from build123d import *

# Parameters (mm, degrees)
SKETCH1_R           = 4.25
SKETCH1_R_2         = 1.25
BOSS_EXTRUDE1_DEPTH = 3
BOSS_EXTRUDE2_START = -3
SKETCH2_R           = 2.5
SKETCH2_R_2         = 1.25
BOSS_EXTRUDE2_DEPTH = 6


with BuildPart() as part:
    # Sketch1 → Boss-Extrude1 (new body)
    # profile 1 of 4: a face of its own
    with BuildSketch(Plane(origin=(0, 0, 0), x_dir=(1, 0, 0), z_dir=(0, 1, 0))):
        with BuildLine():
            ThreePointArc((1.6e-08, -11.5), (-11.5, -2.4e-08), (-3.2e-08, 11.5))
            ThreePointArc((-3.2e-08, 11.5), (-4.157986242, 14.870426004), (-1.721061947, 19.635929204))
            ThreePointArc((-1.721061947, 19.635929204), (-14.5, 0), (-1.721061947, -19.635929204))
            ThreePointArc((-1.721061947, -19.635929204), (-4.157986237, -14.87042598), (1.6e-08, -11.5))
        make_face()
    # profile 2 of 4: a face of its own
    with BuildSketch(Plane(origin=(0, 0, 0), x_dir=(1, 0, 0), z_dir=(0, 1, 0))):
        with BuildLine():
            ThreePointArc((1.721061947, 19.635929204), (3.562093014, 18.068187517), (4.25, 15.75))
            ThreePointArc((4.25, 15.75), (3.005203809, 12.744796169), (-3.2e-08, 11.5))
            ThreePointArc((-3.2e-08, 11.5), (8.131727972, 8.131727995), (11.5, 0))
            ThreePointArc((11.5, 0), (8.131727989, -8.131727978), (1.6e-08, -11.5))
            ThreePointArc((1.6e-08, -11.5), (3.005203826, -12.744796186), (4.25, -15.75))
            ThreePointArc((4.25, -15.75), (3.562093014, -18.068187517), (1.721061947, -19.635929204))
            ThreePointArc((1.721061947, -19.635929204), (14.5, 0), (1.721061947, 19.635929204))
        make_face()
    # profile 3 of 4: a face of its own
    with BuildSketch(Plane(origin=(0, 0, 0), x_dir=(1, 0, 0), z_dir=(0, 1, 0))):
        with Locations((0, 15.75)):
            Circle(SKETCH1_R)
        with Locations(Location((0, 15.75, 0), (0, 0, 270))):
            Circle(SKETCH1_R_2, mode=Mode.SUBTRACT)
    # profile 4 of 4: a face of its own
    with BuildSketch(Plane(origin=(0, 0, 0), x_dir=(1, 0, 0), z_dir=(0, 1, 0))):
        with Locations((0, -15.75)):
            Circle(SKETCH1_R)
        with Locations(Location((0, -15.75, 0), (0, 0, 270))):
            Circle(SKETCH1_R_2, mode=Mode.SUBTRACT)
    extrude(amount=BOSS_EXTRUDE1_DEPTH)

    # Sketch2 → Boss-Extrude2 (add)
    with BuildSketch(Plane(origin=(0, 3, 0), x_dir=(1, 0, 0), z_dir=(0, 1, 0)).offset(BOSS_EXTRUDE2_START)):
        with Locations(Location((0, 15.75, 0), (0, 0, 270))):
            Circle(SKETCH2_R)
        with Locations(Location((0, 15.75, 0), (0, 0, 270))):
            Circle(SKETCH2_R_2, mode=Mode.SUBTRACT)
    boss_extrude2 = extrude(amount=BOSS_EXTRUDE2_DEPTH)

    # Mirror1: Boss-Extrude2 across plane
    add(boss_extrude2.mirror(Plane.XY))


solid = part.part
Here's how the part is built. I have some questions about the finished solid (model axes, mm). A direction names the side the tool comes from. Give positions to 0.01 mm unless a question says otherwise; leave off trailing zeros. Write each loop counter-clockwise with the first axis right and the second up, starting at its lowest first coordinate (ties: lowest second). Pieces come first, ordered by that corner, then holes. Notation, with made-up numbers: (-37, 30) -> (21, 30) arc R17 cw to (21, 51) -> close; hole circle Ø8 at (1, 88.5). An arc over 180 degrees is marked (long way). Use one line per item in the form item = value. Start each with the question number.
1. Imagine slicing it at B-B on z = 2.5. List the corners of the cut face in (x, y) for me, plus the area to 3 significant figures.
2. Imagine slicing it at C-C on x = -0.5. List the corners of the cut face in (y, z) for me.
3. Imagine slicing it at A-A on x = -6.75. List the corners of the cut face in (y, z) for me.
4. If I drill on L1, parallel to X at y = 4.75, z = 15.75; L2, parallel to Y at x = 8, z = -14.5; L3, parallel to Z at x = 1, y = 0.5, over which ranges is the centre line in solid material (lowest first)?
5. Thinking about a two-plate mould opening in X: for faces 1 (the face through (0, 1, 20)), 2 (the face through (11, 3, -5)), 3 (the face through (0, 3, -17)), which applies, +X half, -X half, draft (parallel to the pull), parting line (faces both ways), or undercut?
6. On a 3-axis mill with a long thin cutter (end or side, diameter ignored), from which of +Z, -Z, +X, -X, +Y, -Y can I reach the whole of each face in a straight line? I mean faces 4 (the face through (-1, 6, 17)), 5 (the face through (0.11, 4.479, 18.248)). Say none if no direction works.
7. Imagine slicing it at D-D on z = -15.75. List the corners of the cut face in (x, y) for me, plus the area to 3 significant figures.
8. Will these pins go through, and if not, where does the flat tip stop? pin 1 Ø3 at (x, y) = (10.5, 2.5) entering from -Z; pin 2 Ø5 at (x, z) = (-5.5, -15.5) entering from +Y; pin 3 Ø3 at (y, z) = (4, -3) entering from -X.
Entries:
q1.outline = (-14.35, 0) -> (-11.22, 0) -> (-11.22, 3) -> (-14.35, 3) -> close; (11.22, 0) -> (14.35, 0) -> (14.35, 3) -> (11.22, 3) -> close
q1.area = 18.8 mm²
q2.outline = (0, -19.97) -> (3, -19.97) -> (3, -18.2) -> (6, -18.2) -> (6, -16.9) -> (0, -16.9) -> close; (0, -14.6) -> (6, -14.6) -> (6, -13.3) -> (3, -13.3) -> (3, -11.49) -> (0, -11.49) -> close; (0, 11.49) -> (3, 11.49) -> (3, 13.3) -> (6, 13.3) -> (6, 14.6) -> (0, 14.6) -> close; (0, 16.9) -> (6, 16.9) -> (6, 18.2) -> (3, 18.2) -> (3, 19.97) -> (0, 19.97) -> close
q3.outline = (0, -16.52) -> (3, -16.52) -> (3, -9.31) -> (0, -9.31) -> close; (0, 9.31) -> (3, 9.31) -> (3, 16.52) -> (0, 16.52) -> close
q4.L1 = -2.5 to -1.25, 1.25 to 2.5
q4.L2 = 0 to 3
q4.L3 = -19.88 to -16.5, -15 to -11.46, 11.46 to 15, 16.5 to 19.88
q5.face_1 = parting line
q5.face_2 = draft
q5.face_3 = undercut
q6.face_4 = +Z, -Z, +X, -X, +Y
q6.face_5 = +Y
q7.outline = (-7.62, 0) -> (-1.25, 0) -> (-1.25, 6) -> (-2.5, 6) -> (-2.5, 3) -> (-7.62, 3) -> close; (1.25, 0) -> (7.62, 0) -> (7.62, 3) -> (2.5, 3) -> (2.5, 6) -> (1.25, 6) -> close
q7.area = 45.7 mm²
q8.pin_1 = -14.35
q8.pin_2 = 3
q8.pin_3 = -14.42
